```python
from build123d import *

# Parameters (mm, degrees)
SKETCH1_W           = 1300
SKETCH1_H           = 600
SKETCH1_W_2         = 1117.676372874
SKETCH1_H_2         = 40
BOSS_EXTRUDE1_DEPTH = 20
SKETCH2_W           = 40
SKETCH2_H           = 10
BOSS_EXTRUDE2_DEPTH = 40
SKETCH3_R           = 5
CUT_EXTRUDE1_DEPTH  = 10
SKETCH4_W           = 40
SKETCH4_H           = 10
BOSS_EXTRUDE3_DEPTH = 50
SKETCH5_R           = 5
CUT_EXTRUDE2_DEPTH  = 10


with BuildPart() as part:
    # Sketch1 → Boss-Extrude1 (new body)
    with BuildSketch(Plane.XY):
        Rectangle(SKETCH1_W, SKETCH1_H)
        Rectangle(SKETCH1_W_2, SKETCH1_H_2, mode=Mode.SUBTRACT)
    extrude(amount=BOSS_EXTRUDE1_DEPTH)

    # Sketch2 → Boss-Extrude2 (add)
    with BuildSketch(Plane.XY.offset(20)):
        with Locations((-338.838186437, 25)):
            Rectangle(SKETCH2_W, SKETCH2_H)
        with Locations((-338.838186437, -25)):
            Rectangle(SKETCH2_W, SKETCH2_H)
    extrude(amount=BOSS_EXTRUDE2_DEPTH)

    # Sketch3 → Cut-Extrude1 (cut)
    with BuildSketch(Plane.XZ.offset(30)):
        with Locations((-338.838186437, 40)):
            Circle(SKETCH3_R)
    extrude(amount=-CUT_EXTRUDE1_DEPTH, mode=Mode.SUBTRACT)

    # Sketch4 → Boss-Extrude3 (add)
    with BuildSketch(Plane.XY.offset(60)):
        with Locations((-338.838186437, 25)):
            Rectangle(SKETCH4_W, SKETCH4_H)
    extrude(amount=BOSS_EXTRUDE3_DEPTH)

    # Sketch5 → Cut-Extrude2 (cut)
    with BuildSketch(Plane.XZ.offset(-20)):
        with Locations(Location((-338.838186437, 90, 0), (0, 0, 270))):
            Circle(SKETCH5_R)
    extrude(amount=-CUT_EXTRUDE2_DEPTH, mode=Mode.SUBTRACT)


solid = part.part
```
Check sheet for the modelled part. Datum: model origin and axes. Units: mm. A direction names the side the tool comes from. Give positions to 0.01 mm unless a question says otherwise; leave off trailing zeros. Write each loop counter-clockwise with the first axis right and the second up, starting at its lowest first coordinate (ties: lowest second). Pieces come first, ordered by that corner, then holes.
Item 1: Draft check along X on faces 1 (the face through (-44, 20, 18)), 2 (the face through (-335, -30, 44)). Enter one of: released by +X, released by -X, zero draft, split by the parting line, or undercut.
Item 2: Gauge pin test, flat ends, axial feed: pin 1 (11 mm diameter, centred on y = 23.5, z = 60.5, fed in from -X); pin 2 (8 mm diameter, centred on x = -338.84, z = 40, fed in from -Y); pin 3 (2 mm diameter, centred on x = -248.5, y = -227, fed in from +Z); pin 4 (18 mm diameter, centred on x = 54.5, z = 34.5, fed in from +Y). Record the tip position at first contact, or that the pin passes through.
Item 3: Access from +Z, -Z, +X, -X, +Y, -Y to the whole of each face (thin tool, end or side, straight path). Record for faces 3 (the face through (-44, -20, 14)), 4 (the face through (-9, 71, 0)), 5 (the face through (-339, 30, 64)).
Item 4: Cross-section at B-B (y = 164). Enter the section's corners in (x, z).
Item 5: Cross-section at A-A (x = -181). Enter the section's corners in (y, z).
Item 6: Scan lines: L1, parallel to X at y = 26, z = 90; L2, parallel to Z at x = 358, y = 262.5. Record each from-to range of solid material in increasing order.
Report:
1. face 1: undercut
1. face 2: zero draft
2. pin 1: stops at x = -358.84
2. pin 2: stops at y = 20
2. pin 3: stops at z = 20
2. pin 4: passes through
3. face 3: +Z, -Z
3. face 4: -Z, +X, -X, +Y, -Y
3. face 5: +Z, +X, -X, +Y
4. outline: (-650, 0) - (650, 0) - (650, 20) - (-650, 20) - close
5. outline: (-300, 0) - (-20, 0) - (-20, 20) - (-300, 20) - close; (20, 0) - (300, 0) - (300, 20) - (20, 20) - close
6. L1: x = -358.84 to -343.84, -333.84 to -318.84
6. L2: z = 0 to 20
